Read the model definition and answer for the solid it produces. Units are mm, in the model's axes. Face numbers are marked on the shaded views. Coordinates: 2 decimals unless noted, no trailing zeros. Loops run counter-clockwise (first coordinate to the right, second up) from the corner with the lowest first, then second, coordinate; pieces in that order, holes last. Notation, with made-up numbers: M 70.5,-26.75 L 78.5,-26.75 A35 ccw 78.5,11.25 Z; hole C 9,1.25 d5. An arc over 180 degrees is marked long. Put each result on its own line as item: value.
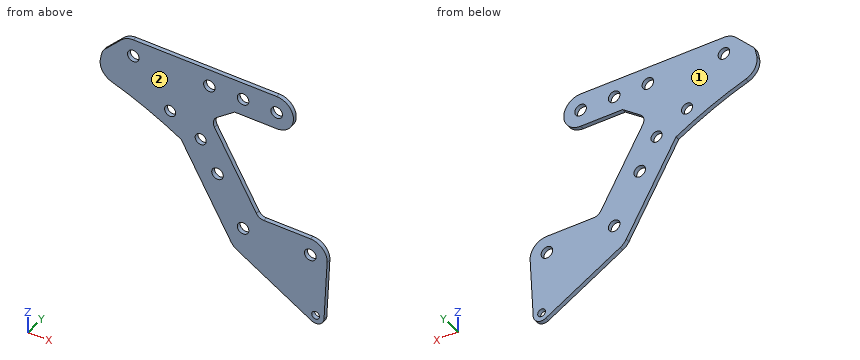
Autodesk Inventor part; units mm, degrees
ref_plane "YZ Plane" through (0, 0, 0) normal (1, 0, 0) x (0, 1, 0)
ref_plane "XZ Plane" through (0, 0, 0) normal (0, 1, 0) x (-1, 0, 0)
ref_plane "XY Plane" through (0, 0, 0) normal (0, 0, 1) x (1, 0, 0)
sketch "main" plane through (0, 0, 0) normal (0, 0, 1) x (1, 0, 0)
  circle A0 centre (36.4896, 64.2776) radius 2.1844
  line L0 (36.4904, 70.6276) -> (-17.6528, 70.6344)
  circle A1 centre (7.7473, 64.2844) radius 2.1844
  line L1 (-17.6416, 57.9344) -> (-1.7768, 57.9386)
  arc A2 (-17.6528, 70.6344) -> (-17.6416, 57.9344) centre (-17.6528, 64.2844) ccw
  circle A3 centre (-17.6528, 64.2844) radius 2.1844
  arc A4 (40.98, 68.7674) -> (36.4904, 70.6276) centre (36.4896, 64.2776) ccw
  line L2 (40.98, 68.7674) -> (49.8505, 68.7674) construction
  circle A5 centre (-4.9416, 13.4844) radius 2.1844
  circle A6 centre (-4.9528, 64.287) radius 2.1844
  point P0 (10.5119, 26.5593)
  point P1 (34.4277, 26.6577)
  dimension "d2" = 4.3688
  dimension "d3" = 4.3688
  dimension "d13" = 6.35
  dimension "d78" = 4.3688
sketch "mogo" plane through (0, 0, 0) normal (0, 0, 1) x (1, 0, 0)
  line L0 (-61.3822, 498.7735) -> (65.6178, 572.097)
  line L1 (65.6178, 572.097) -> (192.6178, 498.7735)
  line L2 (192.6178, 498.7735) -> (192.6178, 352.1265)
  line L3 (192.6178, 352.1265) -> (65.6178, 278.803)
  line L4 (65.6178, 278.803) -> (-61.3822, 352.1265)
  line L5 (-61.3822, 352.1265) -> (-61.3822, 498.7735)
  point P0 (65.6178, 425.45)
  point P1 (65.6178, 425.45)
  dimension "d59" = 254
sketch "Sketch1" plane through (0, 0, 0) normal (0, 1, 0) x (-1, 0, 0)
  line L0 (58.6337, 4.471) -> (65.1127, -2.0089)
  arc A0 (65.935, -3.4345) -> (65.1127, -2.0089) centre (62.8675, -4.2538) ccw
  circle A1 centre (22.3424, -33.2913) radius 2.1844
  arc A2 (66.587, -6.4669) -> (65.935, -3.4345) centre (35.461, -11.5736) ccw
  arc A3 (62.3569, -13.5096) -> (66.587, -6.4669) centre (60.3208, -7.4949) ccw
  line L1 (31.7488, -5.4171) -> (31.751, 4.6095)
  arc A4 (62.3569, -13.5096) -> (36.0563, -25.4131) centre (109.3798, -152.4131) ccw
  line L2 (36.0563, -25.4131) -> (17.2601, -57.9692)
  line L3 (7.6511, -42.8625) -> (23.5038, -15.4048)
  line L4 (49.7771, -4.633) -> (49.6408, -4.4967)
  line L5 (4.9014, -44.45) -> (-12.7, -44.45)
  line L6 (-17.8837, -73.9061) -> (-19.0418, -51.1224)
  line L7 (14.9358, -60.2934) -> (-13.1253, -76.4945)
  circle A5 centre (-12.7, -50.8) radius 2.1844
  arc A6 (-12.7, -44.45) -> (-19.0418, -51.1224) centre (-12.7, -50.8) ccw
  arc A7 (-17.8837, -73.9061) -> (-13.1253, -76.4945) centre (-14.7128, -73.7449) ccw
  circle A8 centre (-14.7128, -73.7449) radius 1.4693
  arc A9 (14.9358, -60.2934) -> (17.2601, -57.9692) centre (11.7608, -54.7942) ccw
  circle A10 centre (28.6924, -22.2928) radius 2.0955
  line L8 (22.62, -11.2484) -> (15.8746, -6.349)
  arc A11 (23.5038, -15.4048) -> (22.62, -11.2484) centre (20.7541, -13.8173) ccw
  circle A12 centre (40.2193, -15.9401) radius 2.0955
  arc A13 (4.9014, -44.45) -> (7.6511, -42.8625) centre (4.9014, -41.275) ccw
  circle A14 centre (54.1423, -0.0179) radius 2.1844
  line L9 (54.1445, 6.3321) -> (0.0013, 6.35)
  circle A15 centre (25.4, -0.0052) radius 2.1844
  line L10 (0.0098, -6.35) -> (15.8746, -6.349)
  arc A16 (0.0013, 6.35) -> (0.0098, -6.35) centre (0, 0) ccw
  circle A17 centre (0, 0) radius 2.1844
  arc A18 (58.6337, 4.471) -> (54.1445, 6.3321) centre (54.1423, -0.0179) ccw
  line L11 (58.6337, 4.471) -> (67.5042, 4.4692) construction
  circle A19 centre (12.7007, -50.8026) radius 2.1844
  circle A20 centre (12.7, 0) radius 2.1844
  point P0 (0, 0)
  point P1 (65.6981, -2.5943)
  point P2 (58.6337, 4.471)
  point P3 (-17.6202, -79.0897)
  point P4 (16.4093, -59.4427)
  point P5 (15.8746, -6.349)
  dimension "d41" = 3.175
  dimension "d54" = 4.3688
  dimension "d60" = 6.35
  dimension "d64" = 15.875
  dimension "d65" = 4.3688
  dimension "d66" = 12.7
  dimension "d67" = 3.175
  dimension "d68" = 6.35
  dimension "d69" = 4.191
  dimension "d70" = 7.9375
  dimension "d71" = 12.7
  dimension "d72" = 7.9375
  dimension "d75" = 3.175
  dimension "d76" = 4.191
  dimension "d77" = 3.175
extrude "Extrusion1" add sketch "Sketch1" along normal blind 1.5875
properties part number "Funnel Gusset Back Improved V2" material "Acetal Resin, White"
1) Find section D-D, the plane z = -38. Write down the section's boundary in (x, y).
Answer list:
outline: M -28.79,0 L -10.46,0 L -10.46,1.59 L -28.79,1.59 Z
2) Find section A-A, the plane x = -12.7. Write down the section's boundary in (y, z), plus the area to 3 significant figures.
Answer list:
outline: M 0,-61.58 L 1.59,-61.58 L 1.59,-52.99 L 0,-52.99 Z; M 0,-48.62 L 1.59,-48.62 L 1.59,-34.12 L 0,-34.12 Z; M 0,-6.35 L 1.59,-6.35 L 1.59,-2.18 L 0,-2.18 Z; M 0,2.18 L 1.59,2.18 L 1.59,6.35 L 0,6.35 Z
area: 49.9 mm^2
3) Determine the mould class of the marked faces 1 and 2 for opening direction Y: released by +Y, released by -Y, zero draft, split by the parting line, or undercut.
Answer list:
face 1: released by +Y
face 2: released by -Y
4) Find section B-B, the plane x = 11.5. Write down the section's boundary in (y, z), plus the area to 3 significant figures.
Answer list:
outline: M 0,-75.56 L 1.59,-75.56 L 1.59,-52.63 L 0,-52.63 Z; M 0,-48.97 L 1.59,-48.97 L 1.59,-44.45 L 0,-44.45 Z
area: 43.6 mm^2
5) Find section C-C, the plane y = 0.25. Count the separate pieces of the cut face and the enclosed holes in it, plus the area to 3 significant figures.
Answer list:
separate pieces: 1
enclosed holes: 10
area: 2,640 mm^2
6) Given pin 1 Ø0.8 at (x, y) = (8, 1) entering from +Z; pin 2 Ø3 at (x, z) = (-28, -20.5) entering from -Y; pin 3 Ø0.5 at (x, y) = (-15, 1) entering from +Z; pin 4 Ø0.8 at (x, y) = (-7.5, 0.5) entering from -Z, each flat-ended and moving along its own axis, determine where each tip first touches the part or whether it passes through.
Answer list:
pin 1: stops at z = -44.45
pin 2: stops at y = 0
pin 3: stops at z = 6.35
pin 4: stops at z = -64.82
7) Straight lines are drawn through the part: line 1 (Z direction, x = -12.7, y = 1.1); line 2 (Z direction, x = -55, y = 1.35); line 3 (Z direction, x = -40, y = 0.25). For each, find the intervals that lie inside material, in ascending order. Write a range as [from, to].
Answer list:
line 1: z = [-61.58, -52.99], [-48.62, -34.12], [-6.35, -2.18], [2.18, 6.35]
line 2: z = [-16.22, -2.03], [1.99, 6.27]
line 3: z = [-23.22, -18.02], [-13.86, 6.34]
